The model under review builds one solid part; all positions refer to its coordinate system, in mm. A direction names the side the tool comes from. Round coordinates to 2 decimals unless told otherwise and drop trailing zeros. Order: outer loops, then holes, each group sorted by start corner. A loop starts at its lowest first (then second) coordinate and runs counter-clockwise, first axis right, second up. Notation, with made-up numbers: M 54,15.5 L 88,15.5 A11 cw 88,34.5 Z; hole C -27,48.5 d3. An arc over 180 degrees is marked long. Use a Markdown table: item, result. Add a question column.
1. To check wall thickness, follow probe 1 along X at (y, z) = (1, 0.2); probe 2 along Y at (x, z) = (72.55, 2.2); probe 3 along X at (y, z) = (24, 1.2). State the ranges of each line that lie inside material, in increasing order.
2. Consider section B-B on z = 0.8. State the section outline as (x, y) points, then the cut area to 3 significant figures.
3. Consider section C-C on x = 47. State the section outline as (y, z) points, then the cut area to 3 significant figures.
4. For faces 5 (the cylindrical face through (-71.55, 0.42, 1.48)), 6 (the flat face through (76, 0, 1)), list the 3-axis set-ups (+Z, -Z, +X, -X, +Y, -Y) from which the entire face can be reached by the end or side of a thin tool; tool diameter is ignored.
5. Consider section A-A on y = 0. State the section outline as (x, z) points, then the cut area to 3 significant figures.
6. The part is to be moulded in two halves that separate along Y. For faces 1 (the cylindrical face through (74.213, 23.361, 1.479)), 2 (the cylindrical face through (74.96, -26.52, 1.48)), 3 (the cylindrical face through (-0.067, -9.992, 1.479)), 4 (the flat face through (1, -12, 0)), say which applies: +Y half, -Y half, draft (parallel to the pull), parting line (faces both ways), or undercut.
7. Consider section D-D on y = -14. State the section outline as (x, z) points, then the cut area to 3 significant figures.
from build123d import *

# Parameters (mm, degrees)
SKETCH_R  = 1.8
PAD_DEPTH = 3


with BuildPart() as part:
    # Sketch → Pad (new body)
    with BuildSketch(Plane.XY):
        with BuildLine():
            Line((-72.55, 27.5), (72.55, 27.5))
            ThreePointArc((76, 24.05), (74.989518, 26.489518), (72.55, 27.5))
            Line((76, 24.05), (76, -24.05))
            ThreePointArc((72.55, -27.5), (74.989518, -26.489518), (76, -24.05))
            Line((72.55, -27.5), (-72.55, -27.5))
            ThreePointArc((-76, -24.05), (-74.989518, -26.489518), (-72.55, -27.5))
            Line((-76, -24.05), (-76, 24.05))
            ThreePointArc((-72.55, 27.5), (-74.989518, 26.489518), (-76, 24.05))
        make_face()
        with Locations((-72.55, -24.05)):
            Circle(SKETCH_R, mode=Mode.SUBTRACT)
        with Locations((-72.55, 24.05)):
            Circle(SKETCH_R, mode=Mode.SUBTRACT)
        with Locations((72.55, 24.05)):
            Circle(SKETCH_R, mode=Mode.SUBTRACT)
        with Locations((72.55, -24.05)):
            Circle(SKETCH_R, mode=Mode.SUBTRACT)
        with BuildLine():
            ThreePointArc((-52.553572, 19), (-71.553572, 0), (-52.553572, -19))
            Line((-52.553572, -19), (-27.553572, -19))
            ThreePointArc((-27.553572, -19), (-8.553572, 0), (-27.553572, 19))
            Line((-52.553572, 19), (-27.553572, 19))
        make_face(mode=Mode.SUBTRACT)
        with BuildLine():
            ThreePointArc((3.026002, 6.967062), (0, 9.993064), (-3.026002, 6.967062))
            Line((-3.026002, 6.967062), (-3.026002, -6.967062))
            ThreePointArc((-3.026002, -6.967062), (0, -9.993064), (3.026002, -6.967062))
            Line((3.026002, 6.967062), (3.026002, -6.967062))
        make_face(mode=Mode.SUBTRACT)
        with BuildLine():
            ThreePointArc((52.553572, -19), (71.553572, 0), (52.553572, 19))
            Line((52.553572, 19), (27.553572, 19))
            ThreePointArc((27.553572, 19), (8.553572, 0), (27.553572, -19))
            Line((52.553572, -19), (27.553572, -19))
        make_face(mode=Mode.SUBTRACT)
    extrude(amount=PAD_DEPTH)


solid = part.part
Answer block:
| question | item | result |
|---|---|---|
| 1 | probe 1 | -76 to -71.53, -8.58 to -3.03, 3.03 to 8.58, 71.53 to 76 |
| 1 | probe 2 | -27.5 to -25.85, -22.25 to 22.25, 25.85 to 27.5 |
| 1 | probe 3 | -76 to -74.35, -70.75 to 70.75, 74.35 to 76 |
| 2 | outline | M -76,-24.05 A3.45 ccw -72.55,-27.5 L 72.55,-27.5 A3.45 ccw 76,-24.05 L 76,24.05 A3.45 ccw 72.55,27.5 L -72.55,27.5 A3.45 ccw -76,24.05 Z; hole C -72.55,-24.05 d3.6; hole C -72.55,24.05 d3.6; hole M -52.55,-19 L -27.55,-19 A19 ccw -27.55,19 L -52.55,19 A19 ccw Z; hole M -3.03,-6.97 A3.03 ccw 3.03,-6.97 L 3.03,6.97 A3.03 ccw -3.03,6.97 Z; hole M 27.55,-19 L 52.55,-19 A19 ccw 52.55,19 L 27.55,19 A19 ccw Z; hole C 72.55,-24.05 d3.6; hole C 72.55,24.05 d3.6 |
| 2 | area | 4,030 mm^2 |
| 3 | outline | M -27.5,0 L -19,0 L -19,3 L -27.5,3 Z; M 19,0 L 27.5,0 L 27.5,3 L 19,3 Z |
| 3 | area | 51.0 mm^2 |
| 4 | face 5 | +Z, -Z |
| 4 | face 6 | +Z, -Z, +X, +Y, -Y |
| 5 | outline | M -76,0 L -71.55,0 L -71.55,3 L -76,3 Z; M -8.55,0 L -3.03,0 L -3.03,3 L -8.55,3 Z; M 3.03,0 L 8.55,0 L 8.55,3 L 3.03,3 Z; M 71.55,0 L 76,0 L 76,3 L 71.55,3 Z |
| 5 | area | 59.8 mm^2 |
| 6 | face 1 | undercut |
| 6 | face 2 | -Y half |
| 6 | face 3 | undercut |
| 6 | face 4 | draft |
| 7 | outline | M -76,0 L -65.4,0 L -65.4,3 L -76,3 Z; M -14.71,0 L 14.71,0 L 14.71,3 L -14.71,3 Z; M 65.4,0 L 76,0 L 76,3 L 65.4,3 Z |
| 7 | area | 152 mm^2 |
